Source: CAD feature listing. Evaluate the final solid. Frame: model axes, mm. A direction names the side the tool comes from. Give positions to 0.01 mm unless a question says otherwise; leave off trailing zeros. Loops run counter-clockwise (first coordinate to the right, second up) from the corner with the lowest first, then second, coordinate; pieces in that order, holes last.
```python
from build123d import *

# Parameters (mm, degrees)
SKETCH1_R           = 50.8
SKETCH1_R_2         = 3.175
BOSS_EXTRUDE1_DEPTH = 19.05


with BuildPart() as part:
    # Sketch1 → Boss-Extrude1 (new body)
    with BuildSketch(Plane(origin=(0, 0, 0), x_dir=(0, 0, -1), z_dir=(1, 0, 0))):
        with Locations(Location((0, 0, 0), (0, 0, 180))):
            Circle(SKETCH1_R)
        with BuildLine():
            Line((0, 38.1), (0, 12.7))
            ThreePointArc((0, 12.7), (-3.924515829, 12.078417757), (-7.464872704, 10.274515829))
            Line((-7.464872704, 10.274515829), (-22.394618112, 30.823547486))
            ThreePointArc((-22.394618112, 30.823547486), (-11.773547486, 36.235253271), (0, 38.1))
        make_face(mode=Mode.SUBTRACT)
        with BuildLine():
            Line((-36.235253271, 11.773547486), (-12.078417757, 3.924515829))
            ThreePointArc((-12.078417757, 3.924515829), (-12.7, 0), (-12.078417757, -3.924515829))
            Line((-12.078417757, -3.924515829), (-36.235253271, -11.773547486))
            ThreePointArc((-36.235253271, -11.773547486), (-38.1, 0), (-36.235253271, 11.773547486))
        make_face(mode=Mode.SUBTRACT)
        with BuildLine():
            Line((-22.394618112, -30.823547486), (-7.464872704, -10.274515829))
            ThreePointArc((-7.464872704, -10.274515829), (-3.924515829, -12.078417757), (0, -12.7))
            Line((0, -12.7), (0, -38.1))
            ThreePointArc((0, -38.1), (-11.773547486, -36.235253271), (-22.394618112, -30.823547486))
        make_face(mode=Mode.SUBTRACT)
        with BuildLine():
            Line((22.394618112, -30.823547486), (7.464872704, -10.274515829))
            ThreePointArc((7.464872704, -10.274515829), (10.274515829, -7.464872704), (12.078417757, -3.924515829))
            Line((12.078417757, -3.924515829), (36.235253271, -11.773547486))
            ThreePointArc((36.235253271, -11.773547486), (30.823547486, -22.394618112), (22.394618112, -30.823547486))
        make_face(mode=Mode.SUBTRACT)
        with BuildLine():
            Line((36.235253271, 11.773547486), (12.078417757, 3.924515829))
            ThreePointArc((12.078417757, 3.924515829), (10.274515829, 7.464872704), (7.464872704, 10.274515829))
            Line((7.464872704, 10.274515829), (22.394618112, 30.823547486))
            ThreePointArc((22.394618112, 30.823547486), (30.823547486, 22.394618112), (36.235253271, 11.773547486))
        make_face(mode=Mode.SUBTRACT)
        with Locations(Location((0, 0, 0), (0, 0, 180))):
            Circle(SKETCH1_R_2, mode=Mode.SUBTRACT)
    extrude(amount=BOSS_EXTRUDE1_DEPTH)


solid = part.part
```
(1) First-contact query: pin 1 (1.5 mm diameter, centred on x = 10, y = 40, fed in from +Z); pin 2 (6 mm diameter, centred on x = 11, y = -18.5, fed in from +Z); pin 3 (1 mm diameter, centred on x = 4.5, z = -16.5, fed in from +Y). Flat tips, straight axial feed; report the tip coordinate or a pass-through.
A:
pin 1: stops at z = 32.25
pin 2: stops at z = 48.38
pin 3: stops at y = 48.21
(2) Section B-B, the plane x = 3.25. Return the cut outline in (y, z) (3 decimals), then the cut area to 3 significant figures.
A:
outline: circle Ø101.6 at (0, 0); hole (-38.1, 0) - (-12.7, 0) arc R12.7 cw to (-10.275, 7.465) - (-30.824, 22.395) arc R38.1 ccw to start; hole (-30.824, -22.395) arc R38.1 ccw to (-11.774, -36.235) - (-3.925, -12.078) arc R12.7 cw to (-10.275, -7.465) - close; hole (-11.774, 36.235) - (-3.925, 12.078) arc R12.7 cw to (3.925, 12.078) - (11.774, 36.235) arc R38.1 ccw to start; hole circle Ø6.35 at (0, 0); hole (3.925, -12.078) - (11.774, -36.235) arc R38.1 ccw to (30.824, -22.395) - (10.275, -7.465) arc R12.7 cw to start; hole (10.275, 7.465) arc R12.7 cw to (12.7, 0) - (38.1, 0) arc R38.1 ccw to (30.824, 22.395) - close
area: 6,050 mm2
(3) Mould query, pull axis Z, two halves, no side actions, for faces 3 (the cylindrical face through (9.39, 45.07, 23.44)), 4 (the cylindrical face through (9.392, 22.53, -30.725)), 5 (the flat face through (0, -1, 11)). Classes: pulls with the +Z half, pulls with the -Z half, needs draft (parallel to the pull), parting line crosses it, or undercut.
A:
face 3: parting line crosses it
face 4: undercut
face 5: needs draft
(4) Reachability of faces 1 (the cylindrical face through (9.39, -36.29, 11.61)), 2 (the flat face through (19.05, -1, 11)) from +Z, -Z, +X, -X, +Y, -Y: full face, straight path, thin tool, end or side. Return the list, or none.
A:
face 1: +X, -X
face 2: +Z, -Z, +X, +Y, -Y
(5) Section A-A, the plane y = 0. Return the cut outline in (x, z) (3 decimals), then the cut area to 3 significant figures.
A:
outline: (0, -50.8) - (19.05, -50.8) - (19.05, -3.175) - (0, -3.175) - close; (0, 3.175) - (19.05, 3.175) - (19.05, 12.7) - (0, 12.7) - close; (0, 38.1) - (19.05, 38.1) - (19.05, 50.8) - (0, 50.8) - close
area: 1,330 mm2
(6) Section D-D, the plane z = 44. Return the cut outline in (x, y).
A:
outline: (0, -25.39) - (19.05, -25.39) - (19.05, 25.39) - (0, 25.39) - close
(7) Ray query, line 1 along Z through (x, y) = (14.75, 15.5); line 2 along Y through (x, z) = (16.25, -18); line 3 along Z through (x, y) = (4.5, -23.5). Return the intervals inside material, ascending.
A:
line 1: z = -48.38 to -34.8, -11.26 to 0, 11.26 to 48.38
line 2: y = -47.5 to -24.77, -5.85 to 5.85, 24.77 to 47.5
line 3: z = -45.04 to -29.99, -17.07 to 0, 17.07 to 45.04
(8) Section C-C, the plane z = -27. Return the cut outline in (x, y).
A:
outline: (0, -43.03) - (19.05, -43.03) - (19.05, -26.88) - (0, -26.88) - close; (0, -8.77) - (19.05, -8.77) - (19.05, 8.77) - (0, 8.77) - close; (0, 26.88) - (19.05, 26.88) - (19.05, 43.03) - (0, 43.03) - close
